Model file for the job. Use its own axes, mm. Face numbers are marked on the shaded views. A direction names the side the tool comes from. Coordinates: 2 decimals unless noted, no trailing zeros. Write each loop counter-clockwise with the first axis right and the second up, starting at its lowest first coordinate (ties: lowest second). Pieces come first, ordered by that corner, then holes.
Q1. Which spindle directions (+Z, -Z, +X, -X, +Y, -Y) get a long thin tool onto all of the face, cutting with end or side? Do the marked faces 1 and 2. Say none if no direction does.
Q2. Band-saw the part on C-C, the plane y = -6.5. Write the cut outline in (x, z).
Q3. Pin check, flat tips, straight feed: P1, Ø3, axis at x = 0, y = -2, coming from the +Z side; P2, Ø3, axis at y = 5.5, z = 8, coming from the -X side; P3, Ø1, axis at y = -6, z = 5, coming from the -X side. Stop position of each tip, or through.
Q4. Band-saw the part on A-A, the plane y = 0. Write the cut outline in (x, z), plus the area to 3 significant figures.
Q5. Pull direction Y, two halves, no side cores. Call the marked faces 3, 4 and 5: released by +Y, released by -Y, zero draft, split by the parting line, or undercut.
Q6. Drill centre lines: probe 1 along X at (y, z) = (2, 9.5); probe 2 along X at (y, z) = (1, 6); probe 3 along Z at (x, y) = (0.5, 2.5). Where is each one in solid material? Low to high.
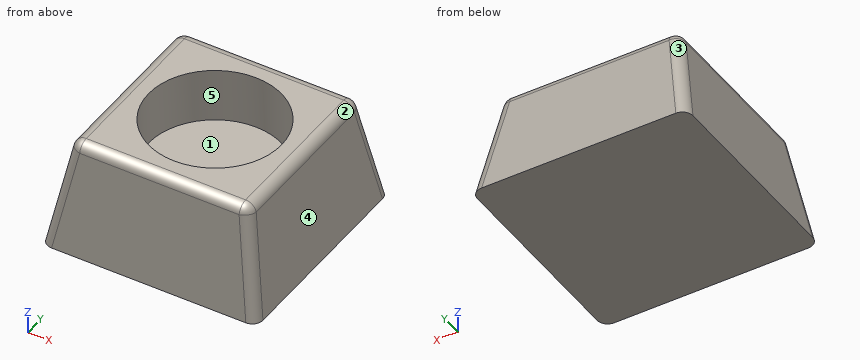
from build123d import *

# Parameters (mm, degrees)
F0_W     = 20
F0_H     = 20
F1_DEPTH = 10
F1_TAPER = 10
F2_R     = 6.173794391
F3_DEPTH = 5
F4_R     = 1


with BuildPart() as f1:
    # F0 (on Top) → F1 (new body)
    with BuildSketch(Plane.XY):
        Rectangle(F0_W, F0_H)
    extrude(amount=F1_DEPTH, taper=F1_TAPER)

    # F2 (on face) → F3 (cut)
    with BuildSketch(Plane.XY.offset(10)):
        Circle(F2_R)
    extrude(amount=-F3_DEPTH, mode=Mode.SUBTRACT)

    # F4
    f4_edges = [f1.edges().sort_by_distance(p)[0] for p in [
        (9.118365, 9.118365, 5),
        (0, 8.23673, 10),
        (8.23673, 0, 10),
        (-9.118365, 9.118365, 5),
        (0, -8.23673, 10),
        (9.118365, -9.118365, 5),
        (-9.118365, -9.118365, 5),
        (-8.23673, 0, 10),
    ]]
    fillet(f4_edges, radius=F4_R)


solid = f1.part
Answer sheet:
1. face 1: +Z
1. face 2: +Z, +X, +Y, -Y
2. outline: (-10, 0) - (10, 0) - (8.38, 9.17) arc R1 ccw to (7.4, 10) - (-7.4, 10) arc R1 ccw to (-8.38, 9.17) - close
3. P1: stops at z = 5
3. P2: stops at x = -8.85
3. P3: stops at x = -9.21
4. outline: (-10, 0) - (10, 0) - (8.38, 9.17) arc R1 ccw to (7.4, 10) - (6.17, 10) - (6.17, 5) - (-6.17, 5) - (-6.17, 10) - (-7.4, 10) arc R1 ccw to (-8.38, 9.17) - close
4. area: 120 mm2
5. face 3: released by +Y
5. face 4: zero draft
5. face 5: undercut
6. probe 1: x = -8.26 to -5.84, 5.84 to 8.26
6. probe 2: x = -8.94 to -6.09, 6.09 to 8.94
6. probe 3: z = 0 to 5
